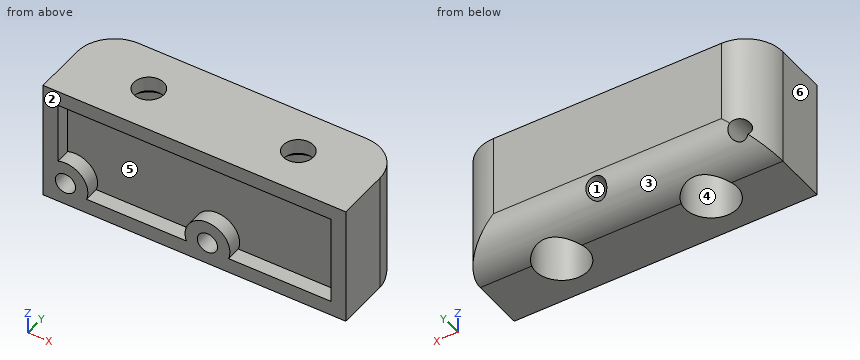
from build123d import *

# Parameters (mm, degrees)
SKETCH1_W           = 40.5
SKETCH1_H           = 16
SKETCH1_R           = 1.35
BOSS_EXTRUDE1_DEPTH = 12
BOSS_EXTRUDE2_START = 2
BOSS_EXTRUDE2_DEPTH = 10
SKETCH2_R           = 3.5
SKETCH2_R_2         = 2
CUT_EXTRUDE1_DEPTH  = 13
SKETCH2_3_R         = 2
CUT_EXTRUDE2_DEPTH  = 29.461596933
CHAMFER1_SIZE       = 1
FILLET1_R           = 5


with BuildPart() as part:
    # Sketch1 → Boss-Extrude1 (new body)
    with BuildSketch(Plane(origin=(0, 0, 0), x_dir=(1, 0, 0), z_dir=(0, 1, 0))):
        Rectangle(SKETCH1_W, SKETCH1_H)
        with Locations(Location((-17.25, 5, 0), (0, 0, 270))):
            Circle(SKETCH1_R, mode=Mode.SUBTRACT)
        with BuildLine():
            Line((-14.421572875, 6), (-1.078427125, 6))
            ThreePointArc((-1.078427125, 6), (1.75, 2), (4.578427125, 6))
            Line((4.578427125, 6), (18.25, 6))
            Line((18.25, 6), (18.25, -6))
            Line((18.25, -6), (-18.25, -6))
            Line((-18.25, -6), (-18.25, 2.171572875))
            ThreePointArc((-18.25, 2.171572875), (-15.128679656, 2.878679656), (-14.421572875, 6))
        make_face(mode=Mode.SUBTRACT)
        with Locations(Location((1.75, 5, 0), (0, 0, 270))):
            Circle(SKETCH1_R, mode=Mode.SUBTRACT)
    extrude(amount=BOSS_EXTRUDE1_DEPTH)

    # Sketch1<3> → Boss-Extrude2 (add)
    with BuildSketch(Plane(origin=(0, 0, 0), x_dir=(1, 0, 0), z_dir=(0, 1, 0)).offset(BOSS_EXTRUDE2_START)):
        with BuildLine():
            ThreePointArc((-14.25, 5), (-15.517949192, 2.550510257), (-18.25, 2.171572875))
            Line((-18.25, 2.171572875), (-18.25, -6))
            Line((-18.25, -6), (18.25, -6))
            Line((18.25, -6), (18.25, 6))
            Line((18.25, 6), (4.578427125, 6))
            ThreePointArc((4.578427125, 6), (4.706795679, 5.507305936), (4.75, 5))
            ThreePointArc((4.75, 5), (1.242694064, 2.043204321), (-1.078427125, 6))
            Line((-1.078427125, 6), (-14.421572875, 6))
            ThreePointArc((-14.421572875, 6), (-14.293204321, 5.507305936), (-14.25, 5))
        make_face()
    extrude(amount=BOSS_EXTRUDE2_DEPTH)

    # Sketch2 → Cut-Extrude1 (cut)
    # profile 1 of 4: a face of its own
    with BuildSketch(Plane(origin=(0, 0, -8), x_dir=(-1, 0, 0), z_dir=(0, 0, -1))):
        with Locations((-10, 6)):
            Circle(SKETCH2_R)
        with Locations((-10, 6)):
            Circle(SKETCH2_R_2, mode=Mode.SUBTRACT)
    # profile 2 of 4: a face of its own
    with BuildSketch(Plane(origin=(0, 0, -8), x_dir=(-1, 0, 0), z_dir=(0, 0, -1))):
        with Locations((-10, 6)):
            Circle(SKETCH2_R_2)
    # profile 3 of 4: a face of its own
    with BuildSketch(Plane(origin=(0, 0, -8), x_dir=(-1, 0, 0), z_dir=(0, 0, -1))):
        with Locations((10, 6)):
            Circle(SKETCH2_R)
        with Locations((10, 6)):
            Circle(SKETCH2_R_2, mode=Mode.SUBTRACT)
    # profile 4 of 4: a face of its own
    with BuildSketch(Plane(origin=(0, 0, -8), x_dir=(-1, 0, 0), z_dir=(0, 0, -1))):
        with Locations((10, 6)):
            Circle(SKETCH2_R_2)
    extrude(amount=-CUT_EXTRUDE1_DEPTH, mode=Mode.SUBTRACT)

    # Sketch2<3> → Cut-Extrude2 (cut, through all)
    with BuildSketch(Plane(origin=(0, 0, -8), x_dir=(-1, 0, 0), z_dir=(0, 0, -1))):
        with Locations((-10, 6)):
            Circle(SKETCH2_3_R)
        with Locations((10, 6)):
            Circle(SKETCH2_3_R)
    extrude(amount=-CUT_EXTRUDE2_DEPTH, mode=Mode.SUBTRACT)

    # Chamfer1
    chamfer1_edges = [part.edges().sort_by_distance(p)[0] for p in [
        (12, 6, 5),
        (-8, 6, 5),
    ]]
    chamfer(chamfer1_edges, length=CHAMFER1_SIZE)

    # Fillet1
    # the kernel refuses this fillet: 5 mm, written as the material it takes off along each edge
    with BuildSketch(Plane(origin=(32.75, 12, -8), x_dir=(0, -1, 0), z_dir=(-1, 0, 0))) as fillet1_piece_1:
        with BuildLine():
            CenterArc((FILLET1_R, FILLET1_R), FILLET1_R, 180, 90)
            Line((0, FILLET1_R), (0, 0))
            Line((0, 0), (FILLET1_R, 0))
        make_face()
    extrude(amount=65.5, mode=Mode.SUBTRACT)
    with BuildSketch(Plane(origin=(20.25, 12, 20.5), x_dir=(0, -1, 0), z_dir=(0, 0, -1))) as fillet1_piece_2:
        with BuildLine():
            CenterArc((FILLET1_R, FILLET1_R), FILLET1_R, 180, 90)
            Line((0, FILLET1_R), (0, 0))
            Line((0, 0), (FILLET1_R, 0))
        make_face()
    extrude(amount=41, mode=Mode.SUBTRACT)
    with BuildSketch(Plane(origin=(-20.25, 12, -20.5), x_dir=(1, 0, 0), z_dir=(0, 0, 1))) as fillet1_piece_3:
        with BuildLine():
            CenterArc((FILLET1_R, -FILLET1_R), FILLET1_R, 90, 90)
            Line((0, -FILLET1_R), (0, 0))
            Line((0, 0), (FILLET1_R, 0))
        make_face()
    extrude(amount=41, mode=Mode.SUBTRACT)


solid = part.part
Source: CAD feature listing. Evaluate the final solid. Frame: model axes, mm. Face numbers are marked on the shaded views. A direction names the side the tool comes from. Round coordinates to 2 decimals unless told otherwise and drop trailing zeros. Loops run counter-clockwise (first coordinate to the right, second up) from the corner with the lowest first, then second, coordinate; pieces in that order, holes last.
Q1. Ray query, line 1 (X direction, y = 6, z = -5); line 2 (Z direction, x = 10, y = 1); line 3 (X direction, y = 5.25, z = 2.75). Return the intervals inside material, ascending.
Q2. Access query for the marked faces 4, 5 and 6. Directions: +Z, -Z, +X, -X, +Y, -Y. A direction counts if a zero-diameter tool reaches every point of the face in a straight line with its end or side. Return the directions, or none.
Q3. Mould query, pull axis Z, two halves, no side actions, for the marked faces 1, 2 and 3. Classes: pulls with the +Z half, pulls with the -Z half, needs draft (parallel to the pull), parting line crosses it, or undercut.
Q4. Section D-D, the plane y = 1.25. Return loops of the section in (x, z).
Q5. First-contact query: P1, Ø2.5, axis at x = 1.75, z = -5, coming from the +Y side; P2, Ø5, axis at x = 10, y = 6, coming from the -Z side; P3, Ø3, axis at x = -14, y = 7.5, coming from the -Z side; P4, Ø3.5, axis at x = -7.5, z = -2.5, coming from the -Y side. Flat tips, straight axial feed; report the tip coordinate or a pass-through.
Q6. Section C-C, the plane z = -0.5. Return loops of the section in (x, y).
Q7. Section B-B, the plane z = -5. Return loops of the section in (x, y), plus the area to 3 significant figures.
Q8. Section A-A, the plane y = 6. Return loops of the section in (x, z), plus the area to 3 significant figures.
Solutions:
1. line 1: x = -20.25 to -18.6, -15.9 to -13.5, -6.5 to 0.4, 3.1 to 6.5, 13.5 to 20.25
1. line 2: z = -8 to -6, 6 to 8
1. line 3: x = -20.25 to -13.42, -6.58 to 6.58, 13.42 to 20.25
2. face 4: -Z
2. face 5: -Y
2. face 6: +Z, -Z, -X, +Y, -Y
3. face 1: undercut
3. face 2: needs draft
3. face 3: pulls with the -Z half
4. outline: (-20.25, -8) - (20.25, -8) - (20.25, 8) - (-20.25, 8) - close; hole circle Ø2.7 at (-17.25, -5); hole (-18.25, -2.17) arc R3 cw to (-14.42, -6) - (-1.08, -6) arc R3 cw (long way) to (4.58, -6) - (18.25, -6) - (18.25, 6) - (-18.25, 6) - close; hole circle Ø2.7 at (1.75, -5)
5. P1: passes through
5. P2: stops at z = 5.5
5. P3: stops at z = -8
5. P4: stops at y = 2
6. outline: (-20.25, 0) - (-18.25, 0) - (-18.25, 2) - (18.25, 2) - (18.25, 0) - (20.25, 0) - (20.25, 7) arc R5 ccw to (15.25, 12) - (-15.25, 12) arc R5 ccw to (-20.25, 7) - close; hole circle Ø7 at (-10, 6); hole circle Ø7 at (10, 6)
7. outline: (-20.25, 0) - (-18.6, 0) - (-18.6, 10.71) arc R5 ccw to (-20.25, 7) - close; (-15.9, 0) - (-14.25, 0) - (-14.25, 2) - (-1.25, 2) - (-1.25, 0) - (0.4, 0) - (0.4, 11.58) - (-15.9, 11.58) - close; (3.1, 0) - (4.75, 0) - (4.75, 2) - (18.25, 2) - (18.25, 0) - (20.25, 0) - (20.25, 7) arc R5 ccw to (17.25, 11.58) - (3.1, 11.58) - close; hole circle Ø7 at (-10, 6); hole circle Ø7 at (10, 6)
7. area: 269 mm2
8. outline: (-20.25, -8) - (-13.5, -8) - (-13.5, 5) - (-13, 5) - (-12, 6) - (-12, 8) - (-20.25, 8) - close; (-8, 6) - (-7, 5) - (-6.5, 5) - (-6.5, -8) - (6.5, -8) - (6.5, 5) - (7, 5) - (8, 6) - (8, 8) - (-8, 8) - close; (12, 6) - (13, 5) - (13.5, 5) - (13.5, -8) - (20.25, -8) - (20.25, 8) - (12, 8) - close; hole circle Ø2.7 at (-17.25, -5); hole circle Ø2.7 at (1.75, -5)
8. area: 429 mm2
